The model under review builds one solid part; all positions refer to its coordinate system, in mm. Round coordinates to 2 decimals unless told otherwise and drop trailing zeros. Write each loop counter-clockwise with the first axis right and the second up, starting at its lowest first coordinate (ties: lowest second). Pieces come first, ordered by that corner, then holes. Notation, with made-up numbers: (-10.75, -38) -> (28.25, -38) arc R17 ccw to (28.25, -29) -> close; hole circle Ø10 at (68, 87). An arc over 180 degrees is marked (long way). Return JSON: item names as keys, results as strings. Group by question number.
1. Take a section at C-C, the plane y = 6. Write out the cut boundary in (x, z).
2. Take a section at A-A, the plane z = 1.55. Write out the cut boundary in (x, y).
3. Clearance check with flat-ended pins moving along their axes: P1, Ø0.9, axis at x = 22, z = 1.5, coming from the -Y side; P2, Ø1.5, axis at y = -31, z = 1.5, coming from the +X side; P3, Ø0.9, axis at y = -30, z = 1, coming from the -X side. State where each tip first meets the part, or that it passes through.
4. Take a section at D-D, the plane x = 20. Write out the cut boundary in (y, z).
5. Take a section at B-B, the plane x = 6. Write out the cut boundary in (y, z), then the cut area to 3 significant figures.
6. For line 1 along Y through (x, z) = (6, 2); line 2 along Y through (x, z) = (7.5, 2.5); line 3 along Y through (x, z) = (20, 1.05), list the stretches that pass through material, from the lowest coordinate up. Write a range as from..to.
Autodesk Inventor part; units mm, degrees
ref_plane "YZ Plane" through (0, 0, 0) normal (1, 0, 0) x (0, 1, 0)
ref_plane "XZ Plane" through (0, 0, 0) normal (0, 1, 0) x (-1, 0, 0)
ref_plane "XY Plane" through (0, 0, 0) normal (0, 0, 1) x (1, 0, 0)
sketch "Sketch1" plane through (0, 0, 0) normal (0, 0, 1) x (1, 0, 0)
  line L0 (12, 23) -> (0, 23)
  line L1 (0, 23) -> (0, 0)
  line L2 (0, 0) -> (12, 0)
  line L3 (12, 0) -> (12, 23)
  line L4 (0, 27.5) -> (5.5, 27.5) construction
  line L5 (6.5, 27.5) -> (12, 27.5) construction
  line L6 (0, -4.5) -> (5.5, -4.5) construction
  line L7 (6.5, -4.5) -> (12, -4.5) construction
  line L8 (-10, 3) -> (-10, 31) construction
  line L9 (25, 31) -> (25, 22) construction
  line L10 (25, 12) -> (25, 3) construction
  circle A0 centre (6, 17) radius 2 construction
  circle A1 centre (6, 17) radius 36.225 construction
  circle A2 centre (6, 17) radius 37.6464 construction
  line L11 (-10, 31) -> (25, 31)
  line L12 (25, 31) -> (25, -29)
  line L13 (25, -29) -> (-10, -29)
  line L14 (-10, -29) -> (-10, 31)
  line L15 (7.5, -29) -> (7.5, 31) construction
  line L16 (-2.5, -29) -> (17.5, -29)
  line L17 (17.5, -29) -> (17.5, -32)
  line L18 (17.5, -32) -> (-2.5, -32)
  line L19 (-2.5, -32) -> (-2.5, -29)
  arc A3 (6.5, -3.804) -> (5.5, -3.804) centre (6, -2.55) ccw construction
  arc A4 (5.5, 26.804) -> (6.5, 26.804) centre (6, 25.55) ccw construction
  circle A5 centre (6, 25.55) radius 1.35
  circle A6 centre (6, -2.55) radius 1.35
  line L20 (12.1, 23.1) -> (-0.1, 23.1)
  line L21 (-0.1, 23.1) -> (-0.1, -0.1)
  line L22 (-0.1, -0.1) -> (12.1, -0.1)
  line L23 (12.1, -0.1) -> (12.1, 23.1)
  point P0 (22, -15.5)
  point P1 (25, -15.5)
  dimension "d0" = 60
  dimension "d1" = 3
  dimension "d2" = 10
  dimension "d3" = 10
  dimension "d4" = 0.1
  dimension "d5" = 0.1
  dimension "d6" = 0.1
  dimension "d7" = 0.1
extrude "Extrusion1" add sketch "Sketch1" along normal blind 3 contours L11 L12 L13 L14 | L13 L17 L18 L19
sketch "Sketch2" plane through (0, 0, 3) normal (0, 0, 1) x (1, 0, 0)
  circle A0 centre (-5, -9.15) radius 1.85
  circle A1 centre (20, -9.15) radius 1.85
  point P0 (0, 0)
extrude "Extrusion2" cut sketch "Sketch2" against normal blind 6.175
properties part number "Camera mount raiser"
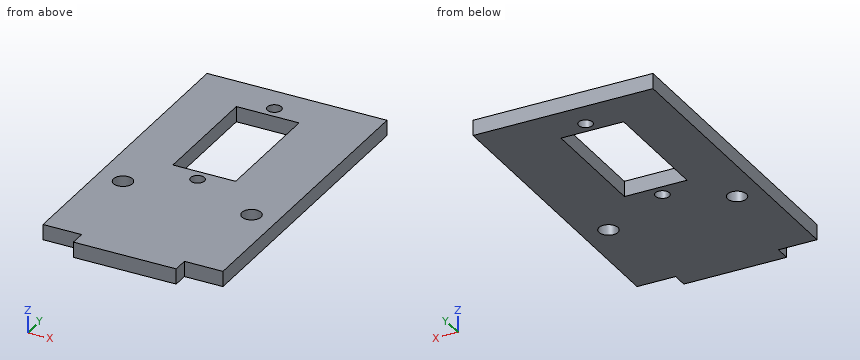
Output:
{
 "1": {"outline": "(-10, 0) -> (-0.1, 0) -> (-0.1, 3) -> (-10, 3) -> close; (12.1, 0) -> (25, 0) -> (25, 3) -> (12.1, 3) -> close"},
 "2": {"outline": "(-10, -29) -> (-2.5, -29) -> (-2.5, -32) -> (17.5, -32) -> (17.5, -29) -> (25, -29) -> (25, 31) -> (-10, 31) -> close; hole circle Ø3.7 at (-5, -9.15); hole (-0.1, -0.1) -> (12.1, -0.1) -> (12.1, 23.1) -> (-0.1, 23.1) -> close; hole circle Ø2.7 at (6, -2.55); hole circle Ø2.7 at (6, 25.55); hole circle Ø3.7 at (20, -9.15)"},
 "3": {"P1": "stops at y = -29", "P2": "stops at x = 17.5", "P3": "stops at x = -2.5"},
 "4": {"outline": "(-29, 0) -> (-11, 0) -> (-11, 3) -> (-29, 3) -> close; (-7.3, 0) -> (31, 0) -> (31, 3) -> (-7.3, 3) -> close"},
 "5": {"outline": "(-32, 0) -> (-3.9, 0) -> (-3.9, 3) -> (-32, 3) -> close; (-1.2, 0) -> (-0.1, 0) -> (-0.1, 3) -> (-1.2, 3) -> close; (23.1, 0) -> (24.2, 0) -> (24.2, 3) -> (23.1, 3) -> close; (26.9, 0) -> (31, 0) -> (31, 3) -> (26.9, 3) -> close", "area": "103 mm^2"},
 "6": {"line 1": "y = -32..-3.9, -1.2..-0.1, 23.1..24.2, 26.9..31", "line 2": "y = -32..-0.1, 23.1..31", "line 3": "y = -29..-11, -7.3..31"}
}
